For this review, take the finished solid that the model builds, in its own axes (mm). A direction names the side the tool comes from. Give positions to 0.01 mm unless a question says otherwise; leave off trailing zeros. Order: outer loops, then holes, each group sorted by start corner. A loop starts at its lowest first (then second) coordinate and runs counter-clockwise, first axis right, second up. Notation, with made-up numbers: (31, 68) - (71, 68) arc R17 cw to (71, 100) - close; hole circle Ø8 at (68, 78). An arc over 180 degrees is marked (long way). One line per item, written item: value.
```python
from build123d import *

# Parameters (mm, degrees)
BOSS_EXTRUDE1_DEPTH = 19.05
SKETCH2_W           = 263.964543074
SKETCH2_H           = 203.2
BOSS_EXTRUDE2_DEPTH = 19.05
SKETCH4_R           = 1.5875
CUT_EXTRUDE1_DEPTH  = 507.449822292
SKETCH5_R           = 1.5875
CUT_EXTRUDE2_DEPTH  = 507.449822292


with BuildPart() as part:
    # Sketch1 → Boss-Extrude1 (new body)
    with BuildSketch(Plane.XY):
        Polygon((-131.982271537, 228.6), (131.982271537, 228.6), (263.964543073, 0), (131.982271537, -228.6), (-131.982271537, -228.6), (-263.964543073, 0), align=None)
    extrude(amount=BOSS_EXTRUDE1_DEPTH)

    # Sketch2 → Boss-Extrude2 (add)
    with BuildSketch(Plane.XY.offset(19.05)):
        with Locations((0, -330.2)):
            Rectangle(SKETCH2_W, SKETCH2_H)
    extrude(amount=-BOSS_EXTRUDE2_DEPTH)

    # Sketch4 → Cut-Extrude1 (cut, through all)
    with BuildSketch(Plane.XY.offset(19.05)):
        Circle(SKETCH4_R)
        with Locations((0, -321.31)):
            Circle(SKETCH4_R)
    extrude(amount=-CUT_EXTRUDE1_DEPTH, mode=Mode.SUBTRACT)

    # Sketch5 → Cut-Extrude2 (cut, through all)
    with BuildSketch(Plane.XY.offset(19.05)):
        with Locations((-121.44375, 0)):
            Circle(SKETCH5_R)
        with Locations((0, 121.44375)):
            Circle(SKETCH5_R)
        with Locations((121.44375, 0)):
            Circle(SKETCH5_R)
        with Locations((0, -121.44375)):
            Circle(SKETCH5_R)
    extrude(amount=-CUT_EXTRUDE2_DEPTH, mode=Mode.SUBTRACT)


solid = part.part
```
(1) Take a section at A-A (z = 15). Write out the cut boundary in (x, y) (1 decimal).
Answers below:
outline: (-264, 0) - (-132, -228.6) - (-132, -431.8) - (132, -431.8) - (132, -228.6) - (264, 0) - (132, 228.6) - (-132, 228.6) - close; hole circle Ø3.2 at (-121.4, 0); hole circle Ø3.2 at (0, -321.3); hole circle Ø3.2 at (0, -121.4); hole circle Ø3.2 at (0, 0); hole circle Ø3.2 at (0, 121.4); hole circle Ø3.2 at (121.4, 0)
(2) Take a section at B-B (y = -336). Write out the cut boundary in (x, z), then the cut area to 3 significant figures.
Answers below:
outline: (-131.98, 0) - (131.98, 0) - (131.98, 19.05) - (-131.98, 19.05) - close
area: 5,030 mm^2
(3) Take a section at C-C (x = 178.5). Write out the cut boundary in (y, z), then the cut area to 3 significant figures.
Answers below:
outline: (-148.03, 0) - (148.03, 0) - (148.03, 19.05) - (-148.03, 19.05) - close
area: 5,640 mm^2
(4) For P1, Ø6, axis at x = 147.5, z = 9, coming from the -Y side; P2, Ø2.5, axis at x = -121.44, y = 0, coming from the -Z side; P3, Ø5.5, axis at y = -357.5, z = 10, coming from the +X side; P4, Ø5, axis at y = 75.5, z = 11, coming from the +X side, all flat-tipped, find the tip position at first contact; note any pin that passes through.
Answers below:
P1: stops at y = -206.92
P2: passes through
P3: stops at x = 131.98
P4: stops at x = 221.82
(5) Machinability: for faces 1 (the face through (131.982, -332, 10)), 2 (the face through (-131.982, -332, 10)), 3 (the face through (-4, -97, 19.05)), which of the approach directions +Z, -Z, +X, -X, +Y, -Y give a long, thin tool a straight path to every point of the face, cutting with its end or side? Answer none if there is none.
Answers below:
face 1: +Z, -Z, +X, -Y
face 2: +Z, -Z, -X, -Y
face 3: +Z, +X, -X, +Y, -Y
(6) Wall thickness on line 1 (Y direction, x = 0, z = 8); line 2 (X direction, y = -321.31, z = 11.25); line 3 (X direction, y = -306, z = 2.5): over which ranges is each line inside the solid? List them lowest first. Write a range as from..to.
Answers below:
line 1: y = -431.8..-322.9, -319.72..-123.03, -119.86..-1.59, 1.59..119.86, 123.03..228.6
line 2: x = -131.98..-1.59, 1.59..131.98
line 3: x = -131.98..131.98
